Autodesk Inventor part; units mm, degrees
ref_plane "conn_XY" through (0, 0, 0) normal (0, 0, -1) x (1, 0, 0)
ref_plane "conn_YZ" through (0, 0, 0) normal (1, 0, 0) x (0, -1, 0)
ref_plane "conn_ZX" through (0, 0, 0) normal (0, -1, 0) x (0, 0, -1)
sketch "Sketch_1" plane through (0, 0, 0) normal (1, 0, 0) x (0, 1, 0)
  line L0 (0, -157.3721) -> (0, 12.7)
  line L1 (0, 12.7) -> (2.634, 12.7)
  line L2 (2.634, 12.7) -> (3.175, 12.159)
  line L3 (3.175, 12.159) -> (3.175, 0)
  line L4 (3.175, 0) -> (4.0005, -0.8255)
  line L5 (4.0005, -0.8255) -> (4.0005, -147.847)
  line L6 (4.0005, -147.847) -> (9.5123, -147.847)
  line L7 (9.5123, -147.847) -> (9.5123, -157.3721)
  line L8 (9.5123, -157.3721) -> (0, -157.3721)
  line L9 (0, -157.3721) -> (0, 12.7)
revolve "Revolution1" add sketch "Sketch_1" angle 360 about axis through (0, 0, -157.3721) along (0, 0, -1)
thread "Thread1"
sketch "Sketch_2" plane through (0, 0, 0) normal (1, 0, 0) x (0, 1, 0)
  line L0 (6.096, 0) -> (3.048, 0)
  line L1 (3.048, 0) -> (3.048, -3.9878)
  line L2 (3.048, -3.9878) -> (6.096, -7.0358)
  line L3 (6.096, -7.0358) -> (6.096, 0)
extrude "Extrusion1" cut sketch "Sketch_2" along normal mid plane 16.002
sketch "Sketch_3" plane through (0, 0, 0) normal (1, 0, 0) x (0, 1, 0)
  line L0 (-6.096, 0) -> (-6.096, -7.0358)
  line L1 (-6.096, -7.0358) -> (-3.048, -3.9878)
  line L2 (-3.048, -3.9878) -> (-3.048, 0)
  line L3 (-3.048, 0) -> (-6.096, 0)
extrude "Extrusion2" cut sketch "Sketch_3" along normal mid plane 16.002
ref_plane "conn_XY" through (0, 0, 0) normal (0, 0, -1) x (1, 0, 0)
ref_plane "conn_YZ" through (0, 0, 0) normal (1, 0, 0) x (0, -1, 0)
ref_plane "conn_ZX" through (0, 0, 0) normal (0, -1, 0) x (0, 0, -1)
properties part number "PR_OCG1-3/4x4" material "Stainless Steel"
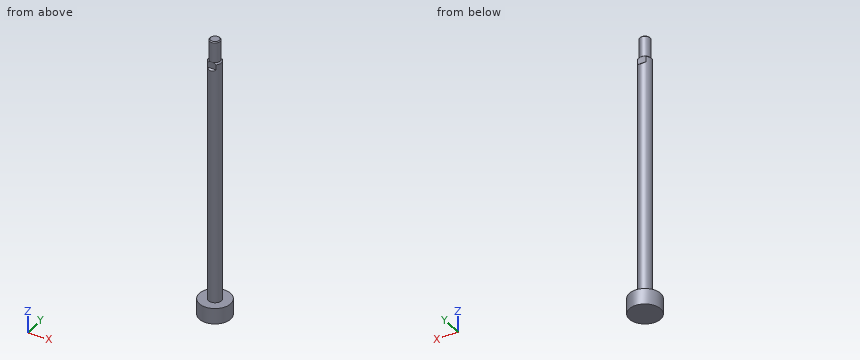
Can you work these out from the model? Positions are in its coordinate system, mm. Round coordinates to 2 decimals unless told otherwise and drop trailing zeros. Order: outer loops, then holes, each group sorted by start corner. A loop starts at its lowest first (then second) coordinate and runs counter-clockwise, first axis right, second up.
(1) If we section it at D-D (y = 7.5): Please give me the cut outline in (x, z), plus the area to 3 significant figures.
Results are:
outline: (-5.85, -157.37) - (5.85, -157.37) - (5.85, -147.85) - (-5.85, -147.85) - close
area: 111 mm2
(2) If I drill on L1, parallel to Y at x = -0.5, z = -75.5; L2, parallel to Z at x = -3.75, y = -7.5; L3, parallel to Y at x = 3, z = -133, over which ranges is the centre line in solid material (lowest first)?
Results are:
L1: y = -3.97 to 3.97
L2: z = -157.37 to -147.85
L3: y = -2.65 to 2.65
(3) I'm going to push flat-ended pins straight in: pin 1 (1.5 mm diameter, centred on x = 0, y = -5.5, fed in from +Z); pin 2 (3 mm diameter, centred on x = -1, z = -3, fed in from +Y); pin 3 (3 mm diameter, centred on y = 0, z = -77, fed in from +X). Where does each tip first touch, or does it pass through?
Results are:
pin 1: stops at z = -147.85
pin 2: stops at y = 3.56
pin 3: stops at x = 4
(4) If we section it at A-A (y = 0): Please give me the cut outline in (x, z) (1 decimal).
Results are:
outline: (-9.5, -157.4) - (9.5, -157.4) - (9.5, -147.8) - (4, -147.8) - (4, -0.8) - (3.2, 0) - (3.2, 12.2) - (2.6, 12.7) - (-2.6, 12.7) - (-3.2, 12.2) - (-3.2, 0) - (-4, -0.8) - (-4, -147.8) - (-9.5, -147.8) - close
(5) If we section it at C-C (x = 7): Please give me the cut outline in (y, z), plus the area to 3 significant figures.
Results are:
outline: (-6.44, -157.37) - (6.44, -157.37) - (6.44, -147.85) - (-6.44, -147.85) - close
area: 123 mm2
(6) If we section it at B-B (z = -67): Please give me the cut outline in (x, y), plus the area to 3 significant figures.
Results are:
outline: circle Ø8 at (0, 0)
area: 50.3 mm2
